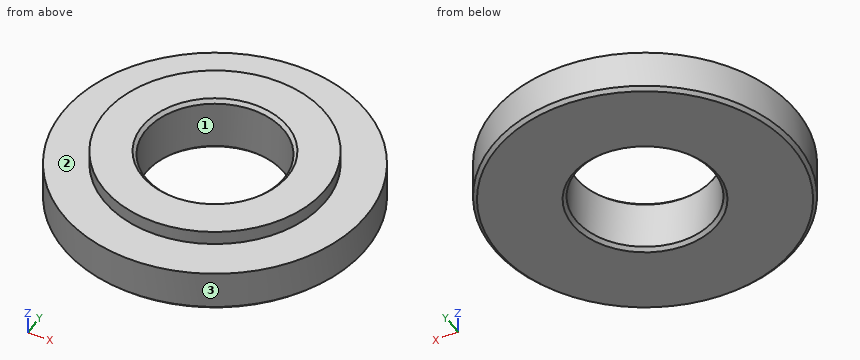
from build123d import *

# Parameters (mm, degrees)
SKETCH017_R     = 10.95
SKETCH017_R_2   = 5
PAD007_DEPTH    = 4
CHAMFER_SIZE    = 0.25
SKETCH023_R     = 10.95
SKETCH023_R_2   = 8
POCKET009_DEPTH = 1


with BuildPart() as part:
    # Sketch017 → Pad007 (new body)
    with BuildSketch(Plane.XY):
        Circle(SKETCH017_R)
        Circle(SKETCH017_R_2, mode=Mode.SUBTRACT)
    extrude(amount=PAD007_DEPTH)

    # Chamfer
    chamfer_edges = [part.edges().sort_by_distance(p)[0] for p in [
        (-10.95, 0, 4),
        (-5, 0, 4),
        (-10.95, 0, 0),
        (-5, 0, 0),
    ]]
    chamfer(chamfer_edges, length=CHAMFER_SIZE)

    # Sketch023 (on Face4 of Pad007) → Pocket009 (cut)
    with BuildSketch(Plane.XY.offset(4)):
        Circle(SKETCH023_R)
        Circle(SKETCH023_R_2, mode=Mode.SUBTRACT)
    extrude(amount=-POCKET009_DEPTH, mode=Mode.SUBTRACT)


solid = part.part
Design review of the part built by this model. Coordinates are the model's own, in mm. Face numbers are marked on the shaded views. Round coordinates to 2 decimals unless told otherwise and drop trailing zeros. Write each loop counter-clockwise with the first axis right and the second up, starting at its lowest first coordinate (ties: lowest second). Pieces come first, ordered by that corner, then holes. Notation, with made-up numbers: (-21, -4) - (22, -4) arc R33 cw to (22, 29) - close; hole circle Ø1 at (-20.5, 39.25). An arc over 180 degrees is marked (long way). Return JSON: item names as keys, results as strings. Group by question number.
Item 1: For probe 1 along Y at (x, z) = (0, 2.8); probe 2 along Z at (x, y) = (-1.5, -9); probe 3 along Y at (x, z) = (3.25, 3.7), list the stretches that pass through material, from the lowest coordinate up. Write a range as [from, to].
Item 2: We need section C-C on z = 2.7. Write out the cut boundary in (x, y), and give its area (3 significant figures).
Item 3: The part is to be moulded in two halves that separate along Y. For the marked faces 1, 2 and 3, say which applies: pulls with the +Y half, pulls with the -Y half, needs draft (parallel to the pull), parting line crosses it, or undercut.
Item 4: We need section A-A on y = 0. Write out the cut boundary in (x, z), and give its area (3 significant figures).
Item 5: Insertion check: P1, Ø1.5, axis at x = 1.5, z = 1.5, coming from the +Y side; P2, Ø1.5, axis at y = -7, z = 3, coming from the -X side; P3, Ø1.5, axis at y = 6, z = 3.5, coming from the -X side. Each pin has a flat end and moves straight along its axis. Give the tip position at first contact, or say it passes through.
Model answer:
{
 "1": {"probe 1": "y = [-10.95, -5], [5, 10.95]", "probe 2": "z = [0, 3]", "probe 3": "y = [-7.31, -3.8], [3.8, 7.31]"},
 "2": {"outline": "circle Ø21.9 at (0, 0); hole circle Ø10 at (0, 0)", "area": "298 mm²"},
 "3": {"face 1": "undercut", "face 2": "needs draft", "face 3": "parting line crosses it"},
 "4": {"outline": "(-10.95, 0.25) - (-10.7, 0) - (-5.25, 0) - (-5, 0.25) - (-5, 3.75) - (-5.25, 4) - (-8, 4) - (-8, 3) - (-10.95, 3) - close; (5, 0.25) - (5.25, 0) - (10.7, 0) - (10.95, 0.25) - (10.95, 3) - (8, 3) - (8, 4) - (5.25, 4) - (5, 3.75) - close", "area": "41.5 mm²"},
 "5": {"P1": "stops at y = 10.92", "P2": "stops at x = -8.99", "P3": "stops at x = -9.5"}
}
